Check sheet for the drawn part. Datum: minimum x, y, z corner. Units: mm. A direction names the side the tool comes from. Give positions to 0.01 mm unless a question says otherwise; leave off trailing zeros. Loops run counter-clockwise (first coordinate to the right, second up) from the corner with the lowest first, then second, coordinate; pieces in that order, holes last. Notation, with made-up numbers: (74, 69) - (88, 69) arc R27 cw to (88, 97) - close; hole circle Ø7 at (13, 61). An arc over 180 degrees is marked (long way). Use a Markdown table: item, result. Add a question column.
1. Cross-section at D-D on x = 1.5. Enter the section's corners in (y, z).
2. Cross-section at C-C on y = 5.25. Enter the section's corners in (x, z).
3. Material ranges on L1, parallel to X at y = 11.5, z = 3.5; L2, parallel to Y at x = 6.75, z = 3.25; L3, parallel to Y at x = 2, z = 2, recorded low to high.
4. Cross-section at A-A on x = 16.25. Enter the section's corners in (y, z).
5. Cross-section at B-B on z = 2.75. Enter the section's corners in (x, y), and give its area (3 significant figures).
6. Depth check by flat-ended pin: P1, Ø1.2, axis at y = 1, z = 3.5, coming from the -X side; P2, Ø3, axis at x = 16.5, z = 3.5, coming from the +Y side; P3, Ø2.5, axis at y = 1, z = 2.5, coming from the +X side; P4, Ø1, axis at x = 4.5, y = 18, coming from the +Z side. Enter the tip coordinate at first touch or a pass-through.
7. Set-up check for the marked faces 1, 2, 3, 4 and 5: record each of +Z, -Z, +X, -X, +Y, -Y from which the full face is reachable in a straight line by a thin tool's end or side.
8. Draft check along Y on the marked faces 6, 7 and 8. Enter one of: pulls with the +Y half, pulls with the -Y half, needs draft (parallel to the pull), parting line crosses it, or undercut.
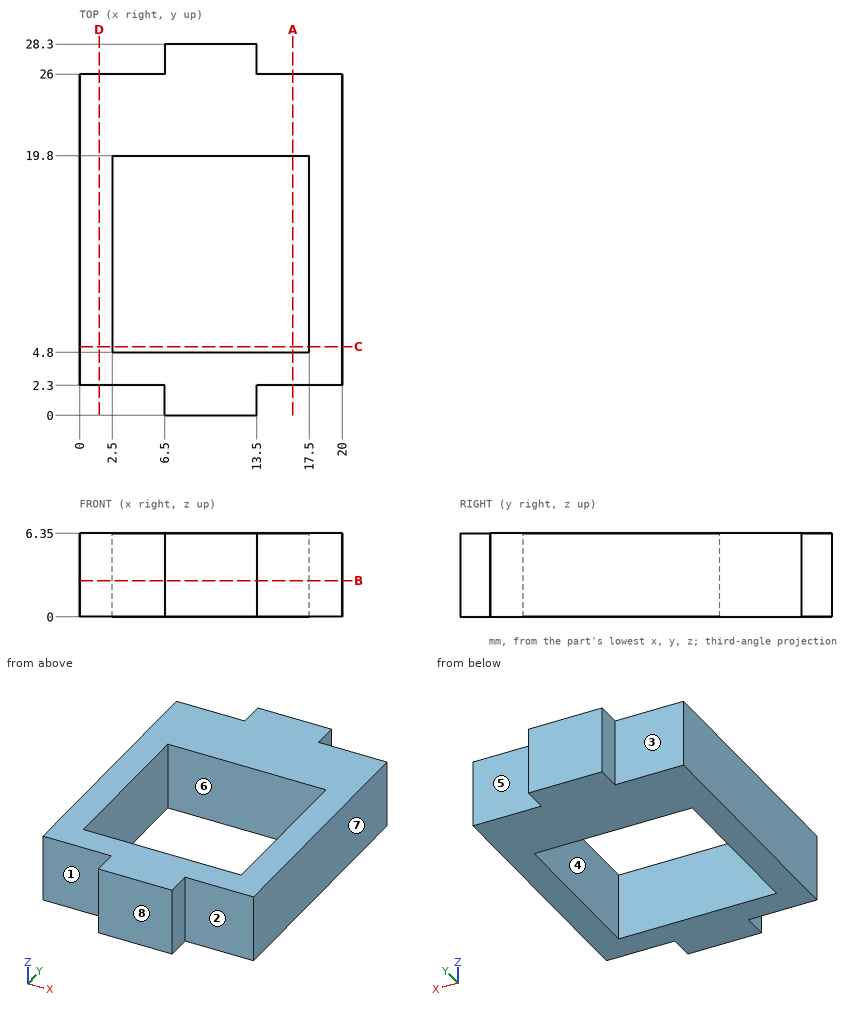
Values found:
| question | item | result |
|---|---|---|
| 1 | outline | (2.3, 0) - (26, 0) - (26, 6.35) - (2.3, 6.35) - close |
| 2 | outline | (0, 0) - (2.5, 0) - (2.5, 6.35) - (0, 6.35) - close; (17.5, 0) - (20, 0) - (20, 6.35) - (17.5, 6.35) - close |
| 3 | L1 | x = 0 to 2.5, 17.5 to 20 |
| 3 | L2 | y = 0 to 4.8, 19.8 to 28.3 |
| 3 | L3 | y = 2.3 to 26 |
| 4 | outline | (2.3, 0) - (4.8, 0) - (4.8, 6.35) - (2.3, 6.35) - close; (19.8, 0) - (26, 0) - (26, 6.35) - (19.8, 6.35) - close |
| 5 | outline | (0, 2.3) - (6.5, 2.3) - (6.5, 0) - (13.5, 0) - (13.5, 2.3) - (20, 2.3) - (20, 26) - (13.5, 26) - (13.5, 28.3) - (6.5, 28.3) - (6.5, 26) - (0, 26) - close; hole (2.5, 4.8) - (17.5, 4.8) - (17.5, 19.8) - (2.5, 19.8) - close |
| 5 | area | 281 mm2 |
| 6 | P1 | stops at x = 6.5 |
| 6 | P2 | stops at y = 26 |
| 6 | P3 | stops at x = 13.5 |
| 6 | P4 | passes through |
| 7 | face 1 | +Z, -Z, -X, -Y |
| 7 | face 2 | +Z, -Z, +X, -Y |
| 7 | face 3 | +Z, -Z, -X, +Y |
| 7 | face 4 | +Z, -Z |
| 7 | face 5 | +Z, -Z, +X, +Y |
| 8 | face 6 | undercut |
| 8 | face 7 | needs draft |
| 8 | face 8 | pulls with the -Y half |
